Read the model definition and answer for the solid it produces. Units are mm, in the model's axes. Face numbers are marked on the shaded views. A direction names the side the tool comes from. Give positions to 0.01 mm unless a question says otherwise; leave off trailing zeros. One line per item, written item: value. Start each with the question number.
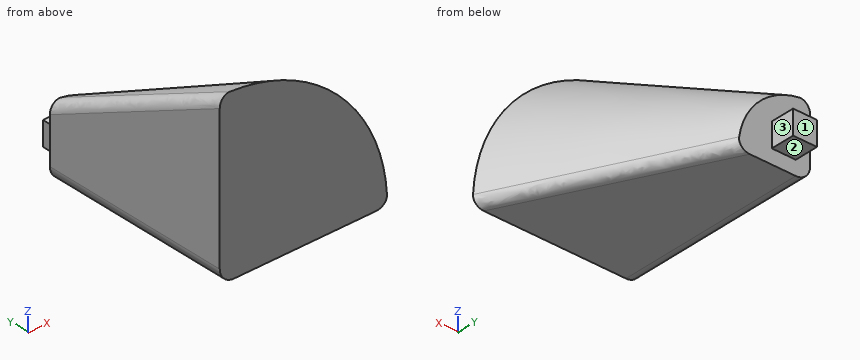
from build123d import *

# Parameters (mm, degrees)
REVOLVE1_ANGLE      = 90
FILLET2_R           = 2
FILLET3_R           = 2
FILLET4_R           = 3
SKETCH2_W           = 5
SKETCH2_H           = 5
BOSS_EXTRUDE1_DEPTH = 5


with BuildPart() as part:
    # Sketch1 → Revolve1 (revolve)
    with BuildSketch(Plane.XY):
        Polygon((0, 0), (15, 0), (35, -40), (0, -40), align=None)
    revolve(axis=Axis((0, 0, 0), (0, -1, 0)), revolution_arc=REVOLVE1_ANGLE)

    # Fillet2
    fillet2_edges = [part.edges().sort_by_distance(p)[0] for p in [
        (0, -20, 25),
    ]]
    fillet(fillet2_edges, radius=FILLET2_R)

    # Fillet3
    fillet3_edges = [part.edges().sort_by_distance(p)[0] for p in [
        (25, -20, 0),
    ]]
    fillet(fillet3_edges, radius=FILLET3_R)

    # Fillet4
    fillet4_edges = [part.edges().sort_by_distance(p)[0] for p in [
        (0, -20, 0),
    ]]
    fillet(fillet4_edges, radius=FILLET4_R)

    # Sketch2 → Boss-Extrude1 (add)
    with BuildSketch(Plane(origin=(0, 0, 0), x_dir=(1, 0, 0), z_dir=(0, 1, 0))):
        with Locations((5.5, -5.5)):
            Rectangle(SKETCH2_W, SKETCH2_H)
    extrude(amount=BOSS_EXTRUDE1_DEPTH)


solid = part.part
Item 1: For the marked faces 1, 2 and 3, determine the directions among +Z, -Z, +X, -X, +Y, -Y from which every point of the face is accessible in a straight line to the end or side of a thin tool.
Item 2: Flat-ended cylindrical pins translate along their axes: pin 1 (5.5 mm diameter, centred on x = 5, y = 3.5, fed in from +Z); pin 2 (6 mm diameter, centred on x = 22.5, z = 11, fed in from +Y); pin 3 (6 mm diameter, centred on y = -33, z = 20.5, fed in from +X). Find the tip coordinate at first contact, or state that the pin passes through.
Item 3: Consider L1, parallel to Y at x = 12.5, z = 5; L2, parallel to Z at x = 9, y = -32; L3, parallel to Y at x = 16, z = 24. Determine where each line is inside the solid, lowest interval first. Write a range as [from, to].
Computed values:
1. face 1: +Z, -Z, +X, -X, +Y
1. face 2: -Z, +X, -X, +Y
1. face 3: +Z, -Z, +X, +Y
2. pin 1: z = 8
2. pin 2: y = -14.09
2. pin 3: x = 26.88
3. L1: [-40, 0]
3. L2: [0, 29.66]
3. L3: [-40, -27.69]
